```python
from build123d import *

# Parameters (mm, degrees)
BOSS_EXTRUDE1_DEPTH                     = 16.5
CUT_EXTRUDE1_REACH                      = 221.937
SKETCH3_W                               = 45
SKETCH3_H                               = 11
FILLET1_R                               = 25
FILLET2_R                               = 10
CUT_EXTRUDE2_REACH                      = 223.786
SKETCH4_R                               = 15
CUT_EXTRUDE3_REACH                      = 223.786
SKETCH5_R                               = 9.75
F_3_0MM_DOWEL_HOLE1_D                   = 3
F_3_0MM_DOWEL_HOLE1_DEPTH               = 19.098709071
F_3_0MM_DOWEL_HOLE1_TIP                 = 0.901290929
CHAMFER1_SIZE                           = 2
CBORE_FOR_M5_HEX_HEAD_BOLT1_D           = 5.5
CBORE_FOR_M5_HEX_HEAD_BOLT1_CBORE_D     = 12.24
CBORE_FOR_M5_HEX_HEAD_BOLT1_CBORE_DEPTH = 3.58


with BuildPart() as part:
    # Sketch1 → Boss-Extrude1 (new, symmetric)
    with BuildSketch(Plane.XY):
        Polygon((0, 0), (-30, 0), (-30, 150), (-90, 150), (-90, 200), (0, 200), align=None)
    extrude(amount=BOSS_EXTRUDE1_DEPTH, both=True)

    # Sketch3 → Cut-Extrude1 (cut, up to next)
    with BuildSketch(Plane(origin=(0, 200, 0), x_dir=(1, 0, 0), z_dir=(0, 1, 0)), mode=Mode.PRIVATE) as cut_extrude1_sk1:
        with Locations((-67.5, 0)):
            Rectangle(SKETCH3_W, SKETCH3_H)
    cut_extrude1_tool1 = extrude(cut_extrude1_sk1.sketch, amount=-CUT_EXTRUDE1_REACH, mode=Mode.PRIVATE) & part.part
    add(cut_extrude1_tool1.solids().sort_by_distance((-67.5, 200, 0))[0], mode=Mode.SUBTRACT)

    # Fillet1
    fillet1_edges = [part.edges().sort_by_distance(p)[0] for p in [
        (0, 200, 0),
    ]]
    fillet(fillet1_edges, radius=FILLET1_R)

    # Fillet2
    fillet2_edges = [part.edges().sort_by_distance(p)[0] for p in [
        (-30, 150, 0),
    ]]
    fillet(fillet2_edges, radius=FILLET2_R)

    # Sketch4 → Cut-Extrude2 (cut, up to next)
    with BuildSketch(Plane.XY.offset(16.5), mode=Mode.PRIVATE) as cut_extrude2_sk1:
        with Locations((-60, 175)):
            Circle(SKETCH4_R)
    cut_extrude2_tool1 = extrude(cut_extrude2_sk1.sketch, amount=-CUT_EXTRUDE2_REACH, mode=Mode.PRIVATE) & part.part
    add(cut_extrude2_tool1.solids().sort_by_distance((-60, 175, 16.5))[0], mode=Mode.SUBTRACT)

    # Sketch5 → Cut-Extrude3 (cut, up to next)
    with BuildSketch(Plane(origin=(0, 0, -16.5), x_dir=(-1, 0, 0), z_dir=(0, 0, -1)), mode=Mode.PRIVATE) as cut_extrude3_sk1:
        with Locations((60, 175)):
            Circle(SKETCH5_R)
    cut_extrude3_tool1 = extrude(cut_extrude3_sk1.sketch, amount=-CUT_EXTRUDE3_REACH, mode=Mode.PRIVATE) & part.part
    add(cut_extrude3_tool1.solids().sort_by_distance((-60, 175, -16.5))[0], mode=Mode.SUBTRACT)

    # Ø3.0mm Dowel Hole1
    with Locations(Plane(origin=(-90, 195, -11), x_dir=(0, 0, -1), z_dir=(-1, 0, 0))):
        with Locations((0, 0), (0, 40), (-22, 0), (-22, 40)):
            Hole(F_3_0MM_DOWEL_HOLE1_D / 2, depth=F_3_0MM_DOWEL_HOLE1_DEPTH)
            with Locations((0, 0, -(F_3_0MM_DOWEL_HOLE1_DEPTH + F_3_0MM_DOWEL_HOLE1_TIP / 2))):  # 118° drill point
                Cone(0, F_3_0MM_DOWEL_HOLE1_D / 2, F_3_0MM_DOWEL_HOLE1_TIP, mode=Mode.SUBTRACT)

    # Chamfer1
    chamfer1_edges = [part.edges().sort_by_distance(p)[0] for p in [
        (-65, 150, -16.5),
        (-57.5, 200, 16.5),
        (-7.32233047, 192.67766953, 16.5),
        (-57.5, 200, -16.5),
        (-7.32233047, 192.67766953, -16.5),
        (-30, 70, 16.5),
        (-30, 70, -16.5),
        (-32.928932188, 147.071067812, 16.5),
        (-32.928932188, 147.071067812, -16.5),
        (0, 87.5, -16.5),
        (-65, 150, 16.5),
        (0, 87.5, 16.5),
    ]]
    chamfer(chamfer1_edges, length=CHAMFER1_SIZE)

    # CBORE for M5 Hex Head Bolt1 (through all)
    with Locations(Plane(origin=(0, 0, 0), x_dir=(0, 0, -1), z_dir=(1, 0, 0))):
        with Locations((0, 10)):
            CounterBoreHole(CBORE_FOR_M5_HEX_HEAD_BOLT1_D / 2, CBORE_FOR_M5_HEX_HEAD_BOLT1_CBORE_D / 2, CBORE_FOR_M5_HEX_HEAD_BOLT1_CBORE_DEPTH)


solid = part.part
```
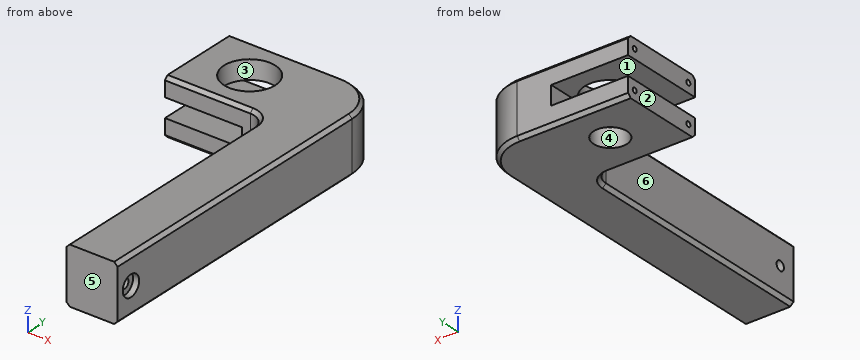
CAD build for the part. Positions are in the model's coordinates, mm. Face numbers are marked on the shaded views. A direction names the side the tool comes from. Coordinates: 2 decimals unless noted, no trailing zeros. Write each loop counter-clockwise with the first axis right and the second up, starting at its lowest first coordinate (ties: lowest second). Pieces come first, ordered by that corner, then holes. Notation, with made-up numbers: (7.5, -19) -> (65.5, -19) arc R27 ccw to (65.5, 1) -> close; hole circle Ø11 at (70, 43.25). An arc over 180 degrees is marked (long way). Return JSON: item names as keys, results as strings. Group by question number.
Q1. Cut at A-A, the plane x = -60. Give the cut face in (y, z).
Q2. Flat gauge pins, fed straight in: pin 1 (5 mm diameter, centred on y = 195, z = -11, fed in from -X); pin 2 (14.5 mm diameter, centred on y = 48.5, z = 7, fed in from -X); pin 3 (5 mm diameter, centred on y = 179, z = 9, fed in from +X); pin 4 (7.5 mm diameter, centred on y = 10, z = 0, fed in from +X). Where does each tip first touch, or does it go through?
Q3. Cut at B-B, the plane z = 0. Give the cut face in (x, y).
Q4. Drill centre lines: line 1 (Y direction, x = -78.25, z = 11); line 2 (Z direction, x = -70.5, y = 157); line 3 (Y direction, x = -71.5, z = 11). Where is each one in solid material? Low to high.
Q5. Pull direction Y, two halves, no side cores. Call the marked faces 4, 5 and 6: released by +Y, released by -Y, zero draft, split by the parting line, or undercut.
Q6. Cut at C-C, the plane y = 75. Give the cut face in (x, z).
Q7. Which spindle directions (+Z, -Z, +X, -X, +Y, -Y) get a long thin tool onto all of the face, cutting with end or side? Do the marked faces 1, 2 and 3. Say none if no direction does.
Returned:
{
 "1": {"outline": "(150, -14.5) -> (152, -16.5) -> (165.25, -16.5) -> (165.25, -5.5) -> (150, -5.5) -> close; (150, 5.5) -> (160, 5.5) -> (160, 16.5) -> (152, 16.5) -> (150, 14.5) -> close; (184.75, -16.5) -> (198, -16.5) -> (200, -14.5) -> (200, -5.5) -> (184.75, -5.5) -> close; (190, 5.5) -> (200, 5.5) -> (200, 14.5) -> (198, 16.5) -> (190, 16.5) -> close"},
 "2": {"pin 1": "stops at x = -90", "pin 2": "stops at x = -30", "pin 3": "stops at x = -0.05", "pin 4": "stops at x = -3.58"},
 "3": {"outline": "(-45, 150) -> (-40, 150) arc R10 cw to (-30, 140) -> (-30, 12.75) -> (-3.58, 12.75) -> (-3.58, 16.12) -> (0, 16.12) -> (0, 175) arc R25 ccw to (-25, 200) -> (-45, 200) -> close; (-30, 0) -> (0, 0) -> (0, 3.88) -> (-3.58, 3.88) -> (-3.58, 7.25) -> (-30, 7.25) -> close"},
 "4": {"line 1": "y = 150 to 153.5, 156.5 to 193.5, 196.5 to 200", "line 2": "z = -16.5 to -5.5, 5.5 to 16.5", "line 3": "y = 150 to 153.5, 156.5 to 165.37, 184.63 to 193.5, 196.5 to 200"},
 "5": {"face 4": "undercut", "face 5": "released by -Y", "face 6": "zero draft"},
 "6": {"outline": "(-30, -14.5) -> (-28, -16.5) -> (-2, -16.5) -> (0, -14.5) -> (0, 14.5) -> (-2, 16.5) -> (-28, 16.5) -> (-30, 14.5) -> close"},
 "7": {"face 1": "-X, +Y, -Y", "face 2": "+Z, -Z, -X, +Y, -Y", "face 3": "+Z"}
}
